Autodesk Inventor part; units mm, degrees
ref_plane "Work Plane3" through (-8.5, 11, 0) normal (1, 0, 0) x (0, 1, 0)
ref_plane "XZ Plane" through (0, 0, 0) normal (0, 1, 0) x (-1, 0, 0)
ref_plane "XY Plane" through (0, 0, 0) normal (0, 0, 1) x (1, 0, 0)
sketch "Sketch1" plane through (0, 0, 0) normal (0, 0, 1) x (1, 0, 0)
  line L0 (0, 0) -> (0, 22)
  line L1 (0, 22) -> (11.5, 22)
  line L2 (11.5, 22) -> (11.5, 21)
  line L3 (11.5, 21) -> (9.5, 21)
  line L4 (9.5, 21) -> (9.5, 1)
  line L5 (9.5, 1) -> (11.5, 1)
  line L6 (11.5, 1) -> (11.5, 0)
  line L7 (11.5, 0) -> (0, 0)
  point P0 (5.75, 0)
  dimension "d0" = 22
  dimension "d1" = 20
  dimension "d2" = 1
  dimension "d3" = 23
  dimension "d4" = 19
revolve "Revolution1" add sketch "Sketch1" angle 360 about axis through (0, 0, 0) along (0, 1, 0)
sketch "Sketch3" plane through (0, 22, 0) normal (0, 1, 0) x (1, 0, 0)
  circle A0 centre (0, 0) radius 8.25
  dimension "d6" = 16.5
extrude "Extrusion1" cut sketch "Sketch3" against normal blind 16
sketch "Sketch4" plane through (0, 0, 0) normal (0, -1, 0) x (1, 0, 0)
  circle A0 centre (0, 0) radius 1.5
  dimension "d9" = 3
extrude "Extrusion2" cut sketch "Sketch4" against normal through all
ref_plane "Work Plane1" through (-9.5, 11, 0) normal (1, 0, 0) x (0, 1, 0)
sketch "Sketch7" plane through (-9.5, 11, 0) normal (1, 0, 0) x (0, 1, 0)
  line L0 (-11, -11.5) -> (-11, 11.5)
  point P0 (-11, 0)
  point P1 (-7.5, 0)
  point P2 (-11, 0)
  dimension "d42" = 3.5
hole "Hole2" at (-9.5, 3.5, 0) direction (-1, 0, 0) diameter 7 end through all
sketch "Sketch8" plane through (-11.5, 0, 0) normal (0, -1, 0) x (1, 0, 0)
  line L0 (6.5, -2.825) -> (9, -2.825)
  line L1 (9, -2.825) -> (9, 2.825)
  line L2 (9, 2.825) -> (6.5, 2.825)
  line L3 (6.5, 2.825) -> (6.5, -2.825)
  circle A0 centre (11.5, 0) radius 9.5
  point P0 (2.235, 2.1)
  point P1 (2.235, -2.1)
  dimension "d58" = 2.5
  dimension "d60" = 2.825
  dimension "d61" = 5.65
  dimension "d62" = 2.5
extrude "Extrusion6" cut sketch "Sketch8" along normal through all both and the other way through all contours L3 L2 L1 L0
ref_plane "Work Plane3" through (-8.5, 11, 0) normal (1, 0, 0) x (0, 1, 0)
sketch "Sketch9" plane through (-8.5, 11, 0) normal (1, 0, 0) x (0, 1, 0)
  point P0 (-11, 0)
  point P1 (-7.5, 0)
hole "Hole3" at (-8.5, 3.5, 0) direction (-1, 0, 0) diameter 7 end through all
hole "Hole4" at (-8.5, 3.5, 0) direction (1, 0, 0) diameter 3.5 depth 8.25 countersink diameter 7 countersink angle 90
properties part number "motor JS2622 jsumo"
Work out the finished part from the listing and answer in its coordinate system (mm). A direction names the side the tool comes from. Give positions to 0.01 mm unless a question says otherwise; leave off trailing zeros. Loops run counter-clockwise (first coordinate to the right, second up) from the corner with the lowest first, then second, coordinate; pieces in that order, holes last. Notation, with made-up numbers: (34.25, 5.25) -> (42.25, 5.25) arc R13 cw to (42.25, 20.25) -> close; hole circle Ø6 at (51, -28). An arc over 180 degrees is marked (long way). Use a Markdown table: item, result. Add a question column.
1) The part is cut by section C-C, the plane y = 15.5. Determine the outline of the cut face in (x, z).
2) Which of the six approach directions +Z, -Z, +X, -X, +Y, -Y give full straight-line access (tool end or side, diameter ignored) to faces 1 (the flat face through (-2.5, 1.7, -0.7)), 2 (the cylindrical face through (7.62, 14.11, 3.16)), 3 (the cylindrical face through (8.776, 10.86, -3.639))?
3) The part is cut by section D-D, the plane z = 5.25. Determine the outline of the cut face in (x, y), plus the area to 3 significant figures.
4) Each of these flat-tipped pins is pushed along its axis until it touches: P1, Ø4, axis at x = -6, y = 13, coming from the +Z side; P2, Ø3, axis at y = 4, z = 0.5, coming from the +X side; P3, Ø4.5, axis at y = 3.5, z = 0, coming from the -X side. Where does it stop, or does it pass through?
5) The part is cut by section B-B, the plane x = 6. Determine the outline of the cut face in (y, z), plus the area to 3 significant figures.
6) The part is cut by section A-A, the plane y = 3.5. Determine the outline of the cut face in (x, z) (3 decimals).
7) Consider line 1 along Y through (x, z) = (8.75, -5.75); line 2 along Z through (x, y) = (0, 1.5); line 3 along Y through (x, z) = (-5.5, 0). Determine where each line is inside the solid, lowest interval first.
8) For a pull along X with two mould halves and no side action, classify faces 4 (the cylindrical face through (-1.5, 21.5, 11.4)), 5 (the flat face through (0, 6, 2)), 6 (the conical face through (-6.859, 1.685, -0.403)), 7 (the flat face through (7, 1, -7)) as +X half, -X half, draft (parallel to the pull), parting line (faces both ways), or undercut.
Reported:
| question | item | result |
|---|---|---|
| 1 | outline | circle Ø19 at (0, 0); hole circle Ø16.5 at (0, 0) |
| 2 | face 1 | +Y, -Y |
| 2 | face 2 | +Y |
| 2 | face 3 | none |
| 3 | outline | (-10.23, 0) -> (10.23, 0) -> (10.23, 1) -> (7.92, 1) -> (7.92, 21) -> (10.23, 21) -> (10.23, 22) -> (6.36, 22) -> (6.36, 6) -> (-6.36, 6) -> (-6.36, 22) -> (-10.23, 22) -> (-10.23, 21) -> (-7.92, 21) -> (-7.92, 1) -> (-10.23, 1) -> close |
| 3 | area | 154 mm^2 |
| 4 | P1 | stops at z = 8.62 |
| 4 | P2 | stops at x = 9.5 |
| 4 | P3 | stops at x = -7.25 |
| 5 | outline | (0, -9.81) -> (1, -9.81) -> (1, -7.37) -> (21, -7.37) -> (21, -9.81) -> (22, -9.81) -> (22, -5.66) -> (6, -5.66) -> (6, 5.66) -> (22, 5.66) -> (22, 9.81) -> (21, 9.81) -> (21, 7.37) -> (1, 7.37) -> (1, 9.81) -> (0, 9.81) -> close |
| 5 | area | 153 mm^2 |
| 6 | outline | (-8.832, -3.5) arc R9.5 ccw (long way) to (-8.832, 3.5) -> (-8.5, 3.5) -> (-6.75, 1.75) -> (-5, 1.75) -> (-5, 2.825) -> (-2.5, 2.825) -> (-2.5, 1.75) -> (-0.25, 1.75) -> (-0.25, 1.479) arc R1.5 cw (long way) to (-0.25, -1.479) -> (-0.25, -1.75) -> (-2.5, -1.75) -> (-2.5, -2.825) -> (-5, -2.825) -> (-5, -1.75) -> (-6.75, -1.75) -> (-8.5, -3.5) -> close |
| 7 | line 1 | y = 0 to 1, 21 to 22 |
| 7 | line 2 | z = -9.5 to -1.5, 1.5 to 9.5 |
| 7 | line 3 | y = 0 to 1.75, 5.25 to 6 |
| 8 | face 4 | parting line |
| 8 | face 5 | undercut |
| 8 | face 6 | -X half |
| 8 | face 7 | draft |
